```python
from build123d import *

# Parameters (mm, degrees)
F0_R          = 4.739513
F1_DEPTH      = 101.6
F1_DEPTH_BACK = 25.4
F3_DEPTH      = 68.875959
F4_W          = 60.299049
F4_H          = 8.607775
F5_DEPTH      = 68.875959


with BuildPart() as f1:
    # F0 (on Right) → F1 (new body, two sides)
    with BuildSketch(Plane.YZ) as f1_sk:
        Polygon((-21.380141, 25.972585), (-40.425949, 25.972585), (-40.425949, -23.252495), (28.44901, -23.252495), (28.44901, 25.972585), (9.403203, 25.972585), (9.403203, 19.771623), (-21.380141, 19.771623), align=None)
        with Locations((-23.484038, -10.747273)):
            Circle(F0_R, mode=Mode.SUBTRACT)
        with Locations((5.995752, -10.747273)):
            Circle(F0_R, mode=Mode.SUBTRACT)
        with Locations((-23.484038, 9.332708)):
            Circle(F0_R, mode=Mode.SUBTRACT)
        with Locations((5.995752, 9.332708)):
            Circle(F0_R, mode=Mode.SUBTRACT)
    extrude(amount=F1_DEPTH)
    extrude(f1_sk.sketch, amount=-F1_DEPTH_BACK)

    # F2 (on face) → F3 (cut, through all)
    with BuildSketch(Plane.XZ.offset(40.425949)):
        Polygon((101.6, 25.972585), (42.277858, 25.972585), (101.6, -23.252495), align=None)
    extrude(amount=-F3_DEPTH, mode=Mode.SUBTRACT)

    # F4 (on face) → F5 (cut, through all)
    with BuildSketch(Plane.XZ.offset(40.425949)):
        with Locations((4.749524, -18.948608)):
            Rectangle(F4_W, F4_H)
    extrude(amount=-F5_DEPTH, mode=Mode.SUBTRACT)


solid = f1.part
```
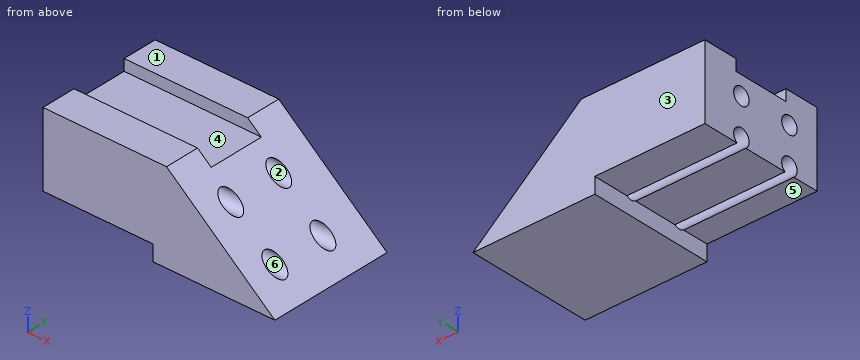
The listing builds one solid part. Answer for the finished solid, in the listing's coordinates (mm). Face numbers are marked on the shaded views. A direction names the side the tool comes from. Coordinates: 2 decimals unless noted, no trailing zeros. Write each loop counter-clockwise with the first axis right and the second up, starting at its lowest first coordinate (ties: lowest second). Pieces come first, ordered by that corner, then holes. Notation, with made-up numbers: (-24.75, 57) - (-16.75, 57) arc R26 cw to (-16.75, 76) - close; hole circle Ø9 at (17, 89.5). An arc over 180 degrees is marked (long way). One line per item, written item: value.
1) Find section D-D (x = -8). Give the vertices of the cut face in (y, z), and give its area (3 significant figures).
Geometry check:
outline: (-40.43, -14.64) - (-26.18, -14.64) arc R4.74 cw (long way) to (-20.79, -14.64) - (3.3, -14.64) arc R4.74 cw (long way) to (8.69, -14.64) - (28.45, -14.64) - (28.45, 25.97) - (9.4, 25.97) - (9.4, 19.77) - (-21.38, 19.77) - (-21.38, 25.97) - (-40.43, 25.97) - close; hole circle Ø9.48 at (-23.48, 9.33); hole circle Ø9.48 at (6, 9.33)
area: 2,330 mm2
2) Find section C-C (x = 39). Give the vertices of the cut face in (y, z), and give its area (3 significant figures).
Geometry check:
outline: (-40.43, -23.25) - (28.45, -23.25) - (28.45, 25.97) - (9.4, 25.97) - (9.4, 19.77) - (-21.38, 19.77) - (-21.38, 25.97) - (-40.43, 25.97) - close; hole circle Ø9.48 at (-23.48, -10.75); hole circle Ø9.48 at (-23.48, 9.33); hole circle Ø9.48 at (6, -10.75); hole circle Ø9.48 at (6, 9.33)
area: 2,920 mm2
3) Find section A-A (z = 6.5). Give the vertices of the cut face in (x, y), and give its area (3 significant figures).
Geometry check:
outline: (-25.4, -40.43) - (65.74, -40.43) - (65.74, -27.28) - (-25.4, -27.28) - close; (-25.4, -19.68) - (65.74, -19.68) - (65.74, 2.2) - (-25.4, 2.2) - close; (-25.4, 9.8) - (65.74, 9.8) - (65.74, 28.45) - (-25.4, 28.45) - close
area: 4,890 mm2
4) For a pull along Y with two mould halves and no side action, classify the marked faces 1, 2 and 3 as pulls with the +Y half, pulls with the -Y half, needs draft (parallel to the pull), parting line crosses it, or undercut.
Geometry check:
face 1: needs draft
face 2: undercut
face 3: pulls with the +Y half
5) Consider line 1 along Y through (x, z) = (55.5, -7.5); line 2 along Y through (x, z) = (13, 23.5); line 3 along Y through (x, z) = (35.5, 5). Determine where each line is inside the solid, lowest interval first. Write a range as from..to.
Geometry check:
line 1: y = -40.43..-26.94, -20.03..2.54, 9.45..28.45
line 2: y = -40.43..-21.38, 9.4..28.45
line 3: y = -40.43..-25.41, -21.56..4.07, 7.92..28.45
6) A tool of negligible diameter and unlimited length cuts with its end or side. For the marked faces 4, 5 and 6, from which of +Z, -Z, +X, -X, +Y, -Y can it reach the whole face along a straight path? Write none if from no direction.
Geometry check:
face 4: +Z, +X, -X
face 5: -Z, -X, +Y, -Y
face 6: +X, -X
7) Find section B-B (y = -9.5). Give the vertices of the cut face in (x, z).
Geometry check:
outline: (-25.4, -14.64) - (34.9, -14.64) - (34.9, -23.25) - (101.6, -23.25) - (49.75, 19.77) - (-25.4, 19.77) - close
8) Each of these flat-tipped pins is pushed along its axis until it touches: pin 1 Ø4.5 at (y, z) = (1.5, -18) entering from -X; pin 2 Ø6 at (x, y) = (58.5, -28) entering from +Z; pin 3 Ø19.5 at (x, y) = (16, -13) entering from -Z; pin 4 Ø5.5 at (y, z) = (-23.48, 9.33) entering from +X. Where does it stop, or does it pass through?
Geometry check:
pin 1: stops at x = 34.9
pin 2: stops at z = 15
pin 3: stops at z = -14.64
pin 4: passes through
